```python
from build123d import *

# Parameters (mm, degrees)
SKETCH_3_R      = 4.562700836
EXTRUDE_3_DEPTH = 38


with BuildPart() as part:
    # 草图3 → 凸台-拉伸3 (new body)
    with BuildSketch(Plane.XY):
        with Locations((92.630544214, 13.494641075)):
            Circle(SKETCH_3_R)
        with BuildLine():
            ThreePointArc((91.130544214, 14.762196375), (92.191204386, 15.201536203), (92.630544214, 16.262196375))
            ThreePointArc((92.630544214, 16.262196375), (92.191204386, 17.322856547), (91.130544214, 17.762196375))
            Line((91.130544214, 17.762196375), (59.64523969, 17.762196375))
            ThreePointArc((59.64523969, 17.762196375), (58.845330036, 17.531111086), (58.291883519, 16.909055768))
            Line((58.291883519, 16.909055768), (55.677790218, 11.439862088))
            ThreePointArc((55.677790218, 11.439862088), (55.124343701, 10.817806769), (54.324434046, 10.586721481))
            Line((54.324434046, 10.586721481), (21.297445186, 10.586721481))
            ThreePointArc((21.297445186, 10.586721481), (20.556052671, 10.390691242), (20.008440624, 9.853837664))
            Line((20.008440624, 9.853837664), (16.684963935, 4.269316435))
            ThreePointArc((16.684963935, 4.269316435), (16.137351889, 3.732462858), (15.395959373, 3.536432619))
            Line((15.395959373, 3.536432619), (1.5, 3.536432619))
            ThreePointArc((1.5, 3.536432619), (0.439339828, 3.09709279), (0, 2.036432619))
            Line((0, 2.036432619), (0, 1.5))
            ThreePointArc((0, 1.5), (0.439339828, 0.439339828), (1.5, 0))
            Line((1.5, 0), (15.415084557, 0))
            ThreePointArc((15.415084557, 0), (16.143809475, 0.188908854), (16.688984275, 0.708053342))
            Line((16.688984275, 0.708053342), (20.004420285, 6.041156217))
            ThreePointArc((20.004420285, 6.041156217), (20.549595084, 6.560300705), (21.278320002, 6.749209559))
            Line((21.278320002, 6.749209559), (54.290974396, 6.749209559))
            ThreePointArc((54.290974396, 6.749209559), (55.110835464, 6.99309339), (55.664095388, 7.645439121))
            Line((55.664095388, 7.645439121), (58.305578349, 13.652814563))
            ThreePointArc((58.305578349, 13.652814563), (58.858838273, 14.305160293), (59.678699341, 14.549044125))
            Line((59.678699341, 14.549044125), (91.130544214, 14.762196375))
        make_face()
    extrude(amount=EXTRUDE_3_DEPTH)


solid = part.part
```
Part model, mm, in its own coordinate system. A direction names the side the tool comes from. Round coordinates to 2 decimals unless told otherwise and drop trailing zeros. Order: outer loops, then holes, each group sorted by start corner. A loop starts at its lowest first (then second) coordinate and runs counter-clockwise, first axis right, second up. Notation, with made-up numbers: M 49,-11.75 L 56,-11.75 A16 ccw 56,-4.75 Z; hole C -34,-8 d3. An arc over 180 degrees is marked long. Answer in a Markdown table with one row per item. Add a question column.
Q1. Wall check: L1, parallel to X at y = 11.25, z = 10; L2, parallel to X at y = 12, z = 5; L3, parallel to Y at x = 30.5, z = 24. Give the ranges that are in metal, low to high. Write a range as from..to.
Q2. 3-axis set-ups, long thin cutter, end or side, ignore diameter. For faces 4 (the face through (52, 10, 38)), 5 (the face through (56.966, 10.607, 18.734)), 6 (the face through (76, 17.762, 19)): which of +Z, -Z, +X, -X, +Y, -Y reach the whole face in a straight line?
Q3. Cut at B-B on x = 26. Give the cut face in (y, z).
Q4. Pin check, flat tips, straight feed: pin 1 (4 mm diameter, centred on x = 10.5, z = 17, fed in from +Y); pin 2 (3 mm diameter, centred on x = 86, z = 12.5, fed in from -Y); pin 3 (10 mm diameter, centred on x = 79.5, z = 25.5, fed in from +Y). Stop position of each tip, or through.
Q5. Mould opens along X. For faces 1 (the face through (95.87, 10.28, 18.73)), 2 (the face through (57, 14.21, 18.73)), 3 (the face through (38, 6.749, 19)) say: +X half, -X half, draft (parallel to the pull), parting line (faces both ways), or undercut.
Q6. Cut at C-C on x = 61.5. Give the cut face in (y, z), and give its area (3 significant figures).
Q7. Cut at A-A on z = 28. Give the cut face in (x, y), and give its area (3 significant figures).
Established:
| question | item | result |
|---|---|---|
| 1 | L1 | x = 55.57..57.25, 88.66..96.6 |
| 1 | L2 | x = 55.95..57.58, 88.32..96.94 |
| 1 | L3 | y = 6.75..10.59 |
| 2 | face 4 | +Z, +X, -X, +Y, -Y |
| 2 | face 5 | +Z, -Z, -Y |
| 2 | face 6 | +Z, -Z, -X, +Y |
| 3 | outline | M 6.75,0 L 10.59,0 L 10.59,38 L 6.75,38 Z |
| 4 | pin 1 | stops at y = 3.54 |
| 4 | pin 2 | stops at y = 14.72 |
| 4 | pin 3 | stops at y = 17.76 |
| 5 | face 1 | undercut |
| 5 | face 2 | -X half |
| 5 | face 3 | draft |
| 6 | outline | M 14.56,0 L 17.76,0 L 17.76,38 L 14.56,38 Z |
| 6 | area | 122 mm2 |
| 7 | outline | M 0,1.5 A1.5 ccw 1.5,0 L 15.42,0 A1.5 ccw 16.69,0.71 L 20,6.04 A1.5 cw 21.28,6.75 L 54.29,6.75 A1.5 ccw 55.66,7.65 L 58.31,13.65 A1.5 cw 59.68,14.55 L 88.24,14.74 A4.56 ccw long 91.02,17.76 L 59.65,17.76 A1.5 ccw 58.29,16.91 L 55.68,11.44 A1.5 cw 54.32,10.59 L 21.3,10.59 A1.5 ccw 20.01,9.85 L 16.68,4.27 A1.5 cw 15.4,3.54 L 1.5,3.54 A1.5 ccw 0,2.04 Z |
| 7 | area | 378 mm2 |
